Check sheet for the modelled part. Datum: model origin and axes. Units: mm. Coordinates: 2 decimals unless noted, no trailing zeros.
Autodesk Inventor part; units mm, degrees
ref_plane "YZ Plane" through (0, 0, 0) normal (1, 0, 0) x (0, 1, 0)
ref_plane "XZ Plane" through (0, 0, 0) normal (0, 1, 0) x (-1, 0, 0)
ref_plane "XY Plane" through (0, 0, 0) normal (0, 0, 1) x (1, 0, 0)
sketch "스케치1" plane through (0, 0, 0) normal (0, 1, 0) x (-1, 0, 0)
  line L0 (-5.3697, -35.4212) -> (-5.3697, -37.6212)
  line L1 (-5.3697, -37.6212) -> (-10.5697, -37.6212)
  line L2 (-10.5697, -37.6212) -> (-10.5697, -35.4212)
  line L3 (-10.5697, -35.4212) -> (-5.3697, -35.4212)
  line L4 (10.6803, 36.7788) -> (10.6803, 38.9788)
  line L5 (10.6803, 38.9788) -> (14.7303, 38.9788)
  line L6 (14.7303, 38.9788) -> (14.7303, 36.7788)
  line L7 (14.7303, 36.7788) -> (10.6803, 36.7788)
  line L8 (14.7303, -35.4212) -> (14.7303, -37.6212)
  line L9 (14.7303, -37.6212) -> (9.5303, -37.6212)
  line L10 (9.5303, -37.6212) -> (9.5303, -35.4212)
  line L11 (9.5303, -35.4212) -> (14.7303, -35.4212)
  line L12 (-5.3697, 36.7788) -> (-10.5697, 36.7788)
  line L13 (-10.5697, 36.7788) -> (-10.5697, 38.9788)
  line L14 (-10.5697, 38.9788) -> (-5.3697, 38.9788)
  line L15 (-5.3697, 38.9788) -> (-5.3697, 36.7788)
  circle A0 centre (12.1303, -19.4212) radius 1.45
  circle A1 centre (-7.9697, -19.4212) radius 1.45
  circle A2 centre (12.1303, 20.7788) radius 1.45
  circle A3 centre (-7.9697, 20.7788) radius 1.45
  line L16 (22.1803, -39.5212) -> (-18.0197, -39.5212)
  line L17 (22.1803, 40.8788) -> (22.1803, -39.5212)
  line L18 (-18.0197, 40.8788) -> (22.1803, 40.8788)
  line L19 (-18.0197, -39.5212) -> (-18.0197, 40.8788)
  line L20 (-27.9197, 50.6788) -> (32.0803, 50.6788)
  line L21 (32.0803, 50.6788) -> (32.0803, -49.3212)
  line L22 (32.0803, -49.3212) -> (-27.9197, -49.3212)
  line L23 (-27.9197, -49.3212) -> (-27.9197, 50.6788)
  line L24 (-27.9197, 50.6788) -> (32.0803, -49.3212) construction
  line L25 (32.0803, 50.6788) -> (-27.9197, -49.3212) construction
  circle A4 centre (12.1303, -19.4212) radius 1.35
  circle A5 centre (-7.9697, -19.4212) radius 1.35
  circle A6 centre (-7.9697, 20.7788) radius 1.35
  circle A7 centre (12.1303, 20.7788) radius 1.35
  circle A8 centre (2.0803, 0.6788) radius 4.7553
  point P0 (0, 0)
  dimension "d0" = 60
  dimension "d1" = 100
  dimension "d4" = 2.7
  dimension "d5" = 2.7
  dimension "d6" = 2.7
  dimension "d7" = 2.7
extrude "돌출1" add sketch "스케치1" along normal blind 6 contours L0 L1 L2 L3 | L4 L5 L6 L7 | L8 L9 L10 L11 | L12 L13 L14 L15 | A0 | A1 | A2 | A3 | L16 L19 L18 L17 | L20 L21 L22 L23 | A4 | A5 | A6 | A7 | A8
sketch "스케치2" plane through (0, 6, 0) normal (0, 1, 0) x (1, 0, 0)
  line L0 (27.9197, 49.3212) -> (-32.0803, 49.3212)
  line L1 (-32.0803, 49.3212) -> (-32.0803, -50.6788)
  line L2 (-32.0803, -50.6788) -> (27.9197, -50.6788)
  line L3 (27.9197, -50.6788) -> (27.9197, 49.3212)
  line L4 (58.4667, -26.0223) -> (58.4667, -28.2223)
  line L5 (58.4667, -28.2223) -> (53.2667, -28.2223)
  line L6 (53.2667, -28.2223) -> (53.2667, -26.0223)
  line L7 (53.2667, -26.0223) -> (58.4667, -26.0223)
  circle A0 centre (15.0977, -21.818) radius 1.45
  circle A1 centre (-5.0023, -21.818) radius 1.45
  line L8 (73.3667, -26.0223) -> (78.5667, -26.0223)
  line L9 (78.5667, -26.0223) -> (78.5667, -28.2223)
  line L10 (73.3667, -28.2223) -> (73.3667, -26.0223)
  line L11 (78.5667, -28.2223) -> (73.3667, -28.2223)
  line L12 (86.0167, -30.1223) -> (45.8167, -30.1223)
  line L13 (74.5167, 46.1777) -> (74.5167, 48.3777)
  line L14 (74.5167, 48.3777) -> (78.5667, 48.3777)
  line L15 (78.5667, 48.3777) -> (78.5667, 46.1777)
  line L16 (45.8167, -30.1223) -> (45.8167, 50.2777)
  line L17 (86.0167, 50.2777) -> (86.0167, -30.1223)
  circle A2 centre (-5.0023, 18.382) radius 1.45
  circle A3 centre (15.0977, 18.382) radius 1.45
  line L18 (58.4667, 46.1777) -> (53.2667, 46.1777)
  line L19 (45.8167, 50.2777) -> (86.0167, 50.2777)
  line L20 (53.2667, 46.1777) -> (53.2667, 48.3777)
  line L21 (53.2667, 48.3777) -> (58.4667, 48.3777)
  line L22 (58.4667, 48.3777) -> (58.4667, 46.1777)
  line L23 (78.5667, 46.1777) -> (74.5167, 46.1777)
  line L24 (-26.6842, 49.3212) -> (33.3158, 49.3212)
  line L25 (33.3158, 49.3212) -> (33.3158, -50.6788)
  line L26 (33.3158, -50.6788) -> (-26.6842, -50.6788)
  line L27 (-26.6842, -50.6788) -> (-26.6842, 49.3212)
  line L28 (-26.6842, 49.3212) -> (33.3158, -50.6788) construction
  line L29 (33.3158, 49.3212) -> (-26.6842, -50.6788) construction
  circle A4 centre (15.0977, -21.818) radius 1.35
  circle A5 centre (-5.0023, -21.818) radius 1.35
  circle A6 centre (-5.0023, 18.382) radius 1.35
  circle A7 centre (15.0977, 18.382) radius 1.35
  circle A8 centre (3.3158, -0.6788) radius 4.7553
  circle A9 centre (-2.0803, -0.6788) radius 10.0549
  line L30 (-6.7392, -0.6788) -> (3.3158, -0.6788)
  point P0 (0, 0)
  point P1 (2.9674, -2.3969)
  dimension "d8" = 60
  dimension "d9" = 100
  dimension "d10" = 2.7
  dimension "d11" = 2.7
  dimension "d12" = 2.7
  dimension "d13" = 2.7
extrude "돌출2" cut sketch "스케치2" against normal blind 6 contours A0 | A2 | A3 | A4 | A5 | A6 | A7
properties part number "feet" material "PMMA 플라스틱"
(1) Go/stop test with a flat-tipped pin: P1, Ø2.5, axis at x = -5, z = 21.82, coming from the -Y side. Record where the tip stops, or that it passes through.
Filled in:
P1: passes through
(2) Thickness scan on probe 1 along X at (y, z) = (1.8, 22); probe 2 along X at (y, z) = (2.1, -18); probe 3 along Z at (x, y) = (16, 0.75). Record the ranges inside material, lowest first.
Filled in:
probe 1: x = -32.08 to -6.34, -3.66 to 13.66, 16.54 to 27.92
probe 2: x = -32.08 to -6.4, -3.6 to 13.7, 16.5 to 27.92
probe 3: z = -49.32 to -19.52, -17.25 to 20.68, 22.95 to 50.68
(3) Release check for a two-part mould opening along X. For faces 1 (the flat face through (-32.08, 3, 1)), 2 (the cylindrical face through (-6.071, 3.042, -19.362)), 3 (the flat face through (-2, 6, 1)), 4 (the flat face through (27.92, 3, 0)) record: +X half, -X half, draft (parallel to the pull), parting line (faces both ways), or undercut.
Filled in:
face 1: -X half
face 2: undercut
face 3: draft
face 4: +X half
